Could you check a few things on this model? Use its own coordinates, in mm. Round coordinates to 2 decimals unless told otherwise and drop trailing zeros. Loops run counter-clockwise (first coordinate to the right, second up) from the corner with the lowest first, then second, coordinate; pieces in that order, holes last. Notation, with made-up numbers: (10.5, 72.5) -> (69.5, 72.5) arc R9 ccw to (69.5, 84.5) -> close; hole circle Ø10 at (-7.5, 85). An arc over 180 degrees is marked (long way). Put each result on its own line as item: value. Start each with the question number.
1. Imagine slicing it at B-B, the plane y = -54.75. Please give me the cut outline in (x, z).
2. Imagine slicing it at C-C, the plane x = -72.75. Please give me the cut outline in (y, z), and give its area (4 significant figures).
3. I'm going to push a flat-ended pin straight in: P1, Ø3.5, axis at x = 67.375, y = 16, coming from the +Z side. Where does the tip first touch, or does it pass through?
4. I need wall thicknesses on line 1 (Y direction, x = -12.5, z = -0.3); line 2 (X direction, y = -59, z = -0.6); line 3 (X direction, y = -50, z = -0.2). Which ranges of each line are inside material? Lowest first, please. Write a range as [from, to].
5. Imagine slicing it at A-A, the plane y = -24.75. Please give me the cut outline in (x, z), and give its area (4 significant figures).
6. If we mould it in two halves opening along X, with no side actions, what happens to faces 1 (the flat face through (-1, 1, 0)), 2 (the cylindrical face through (69.16, -17.37, -0.51))? For each: pulls with the +X half, pulls with the -X half, needs draft (parallel to the pull), parting line crosses it, or undercut.
7. Imagine slicing it at D-D, the plane x = -12.75. Please give me the cut outline in (y, z).
```python
from build123d import *

# Parameters (mm, degrees)
SKETCH_2_W             = 205.5
SKETCH_2_H             = 139.5
SM_BASE_FLANGE_1_DEPTH = 1
FILLET_1_R             = 3
HOLE_WIZARD_M31_D      = 3.15
HOLE_WIZARD_M31_DEPTH  = 8.5
HOLE_WIZARD_M31_TIP    = 0.946355475
SKETCH_9_R             = 2.25
CUT_EXTRUDE_3_DEPTH    = 1
CUT_EXTRUDE_4_DEPTH    = 1
SKETCH_8_R             = 8
CUT_EXTRUDE_1_DEPTH    = 10
SKETCH_10_R            = 9.5
CUT_EXTRUDE_2_DEPTH    = 1
FILLET_2_R             = 0.3


# Sheet-metal steps are written as plain solids
with BuildPart() as part:
    # Sketch 2 → Базовая кромка1 (new body)
    with BuildSketch(Plane.XY):
        Rectangle(SKETCH_2_W, SKETCH_2_H)
    extrude(amount=-SM_BASE_FLANGE_1_DEPTH)

    # Скругление1
    fillet_1_edges = [part.edges().sort_by_distance(p)[0] for p in [
        (-102.75, 69.75, -0.5),
        (102.75, 69.75, -0.5),
        (102.75, -69.75, -0.5),
        (-102.75, -69.75, -0.5),
    ]]
    fillet(fillet_1_edges, radius=FILLET_1_R)

    # Сверло под метчик  спиральное M31
    with Locations(Plane(origin=(0, 0, -1), x_dir=(-1, 0, 0), z_dir=(0, 0, -1))):
        with Locations((-98.021320344, 65.021320344), (98.021320344, 65.021320344), (98.021320344, -65.021320344), (-98.021320344, -65.021320344)):
            Hole(HOLE_WIZARD_M31_D / 2, depth=HOLE_WIZARD_M31_DEPTH)
            with Locations((0, 0, -(HOLE_WIZARD_M31_DEPTH + HOLE_WIZARD_M31_TIP / 2))):  # 118° drill point
                Cone(0, HOLE_WIZARD_M31_D / 2, HOLE_WIZARD_M31_TIP, mode=Mode.SUBTRACT)

    # Эскиз9 → Вырез-Вытянуть3 (cut)
    with BuildSketch(Plane(origin=(0, 0, -1), x_dir=(-1, 0, 0), z_dir=(0, 0, -1))):
        with Locations((-67.375, 16)):
            Circle(SKETCH_9_R)
        with Locations((-35.375, 16)):
            Circle(SKETCH_9_R)
        with Locations((-35.375, -16)):
            Circle(SKETCH_9_R)
        with Locations((-67.375, -16)):
            Circle(SKETCH_9_R)
    extrude(amount=-CUT_EXTRUDE_3_DEPTH, mode=Mode.SUBTRACT)

    # Эскиз11 → Вырез-Вытянуть4 (cut)
    with BuildSketch(Plane(origin=(0, 0, -1), x_dir=(-1, 0, 0), z_dir=(0, 0, -1))):
        with BuildLine():
            Line((-68.375, 8.485281374), (-68.375, -8.485281374))
            ThreePointArc((-68.375, -8.485281374), (-70.375, 0), (-68.375, 8.485281374))
        make_face()
        with BuildLine():
            Line((-66.375, 11.66190379), (-66.375, -11.66190379))
            ThreePointArc((-66.375, -11.66190379), (-65.41793276, -12.798282678), (-64.375, -13.856406461))
            Line((-64.375, -13.856406461), (-64.375, 13.856406461))
            ThreePointArc((-64.375, 13.856406461), (-65.41793276, 12.798282678), (-66.375, 11.66190379))
        make_face()
        with BuildLine():
            Line((-52.375, 18.973665961), (-52.375, -18.973665961))
            ThreePointArc((-52.375, -18.973665961), (-53.377807107, -18.894146281), (-54.375, -18.761663039))
            Line((-54.375, -18.761663039), (-54.375, 18.761663039))
            ThreePointArc((-54.375, 18.761663039), (-53.377807107, 18.894146281), (-52.375, 18.973665961))
        make_face()
        with BuildLine():
            Line((-56.375, 18.33030278), (-56.375, -18.33030278))
            ThreePointArc((-56.375, -18.33030278), (-57.384255298, -18.024673388), (-58.375, -17.663521733))
            Line((-58.375, -17.663521733), (-58.375, 17.663521733))
            ThreePointArc((-58.375, 17.663521733), (-57.384255298, 18.024673388), (-56.375, 18.33030278))
        make_face()
        with BuildLine():
            Line((-60.375, 16.733200531), (-60.375, -16.733200531))
            ThreePointArc((-60.375, -16.733200531), (-61.394240791, -16.143568811), (-62.375, -15.491933385))
            Line((-62.375, -15.491933385), (-62.375, 15.491933385))
            ThreePointArc((-62.375, 15.491933385), (-61.394240791, 16.143568811), (-60.375, 16.733200531))
        make_face()
        with BuildLine():
            Line((-40.375, 15.491933385), (-40.375, -15.491933385))
            ThreePointArc((-40.375, -15.491933385), (-41.355759209, -16.143568811), (-42.375, -16.733200531))
            Line((-42.375, -16.733200531), (-42.375, 16.733200531))
            ThreePointArc((-42.375, 16.733200531), (-41.355759209, 16.143568811), (-40.375, 15.491933385))
        make_face()
        with BuildLine():
            Line((-44.375, 17.663521733), (-44.375, -17.663521733))
            ThreePointArc((-44.375, -17.663521733), (-45.365744702, -18.024673388), (-46.375, -18.33030278))
            Line((-46.375, -18.33030278), (-46.375, 18.33030278))
            ThreePointArc((-46.375, 18.33030278), (-45.365744702, 18.024673388), (-44.375, 17.663521733))
        make_face()
        with BuildLine():
            Line((-48.375, 18.761663039), (-48.375, -18.761663039))
            ThreePointArc((-48.375, -18.761663039), (-49.372192893, -18.894146281), (-50.375, -18.973665961))
            Line((-50.375, -18.973665961), (-50.375, 18.973665961))
            ThreePointArc((-50.375, 18.973665961), (-49.372192893, 18.894146281), (-48.375, 18.761663039))
        make_face()
        with BuildLine():
            Line((-38.375, 13.856406461), (-38.375, -13.856406461))
            ThreePointArc((-38.375, -13.856406461), (-37.33206724, -12.798282678), (-36.375, -11.66190379))
            Line((-36.375, -11.66190379), (-36.375, 11.66190379))
            ThreePointArc((-36.375, 11.66190379), (-37.33206724, 12.798282678), (-38.375, 13.856406461))
        make_face()
        with BuildLine():
            Line((-34.375, 8.485281374), (-34.375, -8.485281374))
            ThreePointArc((-34.375, -8.485281374), (-32.375, 0), (-34.375, 8.485281374))
        make_face()
    extrude(amount=-CUT_EXTRUDE_4_DEPTH, mode=Mode.SUBTRACT)

    # Эскиз8 → Вырез-Вытянуть1 (cut)
    with BuildSketch(Plane(origin=(0, 0, -1), x_dir=(-1, 0, 0), z_dir=(0, 0, -1))):
        with Locations((42.75, -54.75)):
            Circle(SKETCH_8_R)
        with Locations((72.75, -54.75)):
            Circle(SKETCH_8_R)
        with Locations((12.75, -54.75)):
            Circle(SKETCH_8_R)
    extrude(amount=-CUT_EXTRUDE_1_DEPTH, mode=Mode.SUBTRACT)

    # Эскиз10 → Вырез-Вытянуть2 (cut)
    with BuildSketch(Plane(origin=(0, 0, -1), x_dir=(-1, 0, 0), z_dir=(0, 0, -1))):
        with Locations((12.75, -24.75)):
            Circle(SKETCH_10_R)
    extrude(amount=-CUT_EXTRUDE_2_DEPTH, mode=Mode.SUBTRACT)

    # Скругление2
    fillet_2_edges = [part.edges().sort_by_distance(p)[0] for p in [
        (34.375, 8.485281374, -0.5),
        (34.375, -8.485281374, -0.5),
        (68.375, -8.485281374, -0.5),
        (68.375, 8.485281374, -0.5),
        (66.375, 11.66190379, -0.5),
        (64.375, 13.856406461, -0.5),
        (64.375, -13.856406461, -0.5),
        (66.375, -11.66190379, -0.5),
        (54.375, 18.761663039, -0.5),
        (52.375, 18.973665961, -0.5),
        (52.375, -18.973665961, -0.5),
        (54.375, -18.761663039, -0.5),
        (58.375, 17.663521733, -0.5),
        (56.375, 18.33030278, -0.5),
        (56.375, -18.33030278, -0.5),
        (58.375, -17.663521733, -0.5),
        (62.375, 15.491933385, -0.5),
        (60.375, 16.733200531, -0.5),
        (60.375, -16.733200531, -0.5),
        (62.375, -15.491933385, -0.5),
        (44.375, -17.663521733, -0.5),
        (46.375, -18.33030278, -0.5),
        (46.375, 18.33030278, -0.5),
        (44.375, 17.663521733, -0.5),
        (40.375, -15.491933385, -0.5),
        (42.375, -16.733200531, -0.5),
        (42.375, 16.733200531, -0.5),
        (40.375, 15.491933385, -0.5),
        (36.375, -11.66190379, -0.5),
        (38.375, -13.856406461, -0.5),
        (38.375, 13.856406461, -0.5),
        (36.375, 11.66190379, -0.5),
        (48.375, -18.761663039, -0.5),
        (50.375, -18.973665961, -0.5),
        (50.375, 18.973665961, -0.5),
        (48.375, 18.761663039, -0.5),
    ]]
    fillet(fillet_2_edges, radius=FILLET_2_R)


solid = part.part
```
Entries:
1. outline: (-102.75, -1) -> (-80.75, -1) -> (-80.75, 0) -> (-102.75, 0) -> close; (-64.75, -1) -> (-50.75, -1) -> (-50.75, 0) -> (-64.75, 0) -> close; (-34.75, -1) -> (-20.75, -1) -> (-20.75, 0) -> (-34.75, 0) -> close; (-4.75, -1) -> (102.75, -1) -> (102.75, 0) -> (-4.75, 0) -> close
2. outline: (-69.75, -1) -> (-62.75, -1) -> (-62.75, 0) -> (-69.75, 0) -> close; (-46.75, -1) -> (69.75, -1) -> (69.75, 0) -> (-46.75, 0) -> close
2. area: 123.5 mm^2
3. P1: through
4. line 1: [-69.75, -62.75], [-46.75, -34.25], [-15.25, 69.75]
4. line 2: [-102.75, -79.53], [-65.97, -49.53], [-35.97, -19.53], [-5.97, 102.75]
4. line 3: [-102.75, -79.19], [-66.31, -49.19], [-36.31, -19.19], [-6.31, 102.75]
5. outline: (-102.75, -1) -> (-22.25, -1) -> (-22.25, 0) -> (-102.75, 0) -> close; (-3.25, -1) -> (102.75, -1) -> (102.75, 0) -> (-3.25, 0) -> close
5. area: 186.5 mm^2
6. face 1: needs draft
6. face 2: undercut
7. outline: (-69.75, -1) -> (-62.75, -1) -> (-62.75, 0) -> (-69.75, 0) -> close; (-46.75, -1) -> (-34.25, -1) -> (-34.25, 0) -> (-46.75, 0) -> close; (-15.25, -1) -> (69.75, -1) -> (69.75, 0) -> (-15.25, 0) -> close
